from build123d import *

# Parameters (mm, degrees)
F0_R      = 10
F1_DEPTH  = 70
F1_TAPER  = -5
F2_R      = 8
F3_R      = 10
F3_R_2    = 7.5
F1_FACE_R = 10
F4_DEPTH  = 25


with BuildPart() as f1:
    # F0 (on Front) → F1 (new body)
    with BuildSketch(Plane.XZ):
        Circle(F0_R)
    extrude(amount=F1_DEPTH, taper=F1_TAPER)

    # F2
    f2_edges = [f1.edges().sort_by_distance(p)[0] for p in [
        (-16.124206, -70, 0),
    ]]
    fillet(f2_edges, radius=F2_R)

    # F3 (on face) + F1_face (on face) → F4 (join)
    with BuildSketch(Plane(origin=(0, 0, 0), x_dir=(-1, 0, 0), z_dir=(0, 1, 0))):
        Circle(F3_R)
        Circle(F3_R_2, mode=Mode.SUBTRACT)
    with BuildSketch(Plane(origin=(0, 0, 0), x_dir=(1, 0, 0), z_dir=(0, 1, 0))):
        Circle(F1_FACE_R)
    extrude(amount=F4_DEPTH)


solid = f1.part
CAD build for the part. Positions are in the model's coordinates, mm. Coordinates: 2 decimals unless noted, no trailing zeros. Loops run counter-clockwise (first coordinate to the right, second up) from the corner with the lowest first, then second, coordinate; pieces in that order, holes last. Notation, with made-up numbers: (-10, 37) - (21, 37) arc R18 ccw to (21, 68) - close; hole circle Ø8 at (81, 5). An arc over 180 degrees is marked (long way). Write item = value, one per line. Start each with the question number.
Q1. Cut at A-A, the plane y = 7. List the corners of the cut face in (x, z).
Q2. Flat gauge pins, fed straight in: pin 1 Ø2 at (y, z) = (-29.5, 1) entering from +X; pin 2 Ø1 at (x, y) = (2.5, -20.5) entering from +Z; pin 3 Ø3 at (x, y) = (-11, -5) entering from +Z. Where does each tip first touch, or does it go through?
Q3. Pull direction Z, two halves, no side cores. Call faces 1 (the cylindrical face through (2.17, 12.32, -9.76)), 2 (the flat face through (0, 25, 0)): pulls with the +Z half, pulls with the -Z half, needs draft (parallel to the pull), parting line crosses it, or undercut.
Q4. Drill centre lines: L1, parallel to Z at x = 0, y = 19; L2, parallel to Y at x = -6, z = -5.5; L3, parallel to X at y = -23.5, z = -10. Where is each one in solid material? Low to high.
Computed:
q1.outline = circle Ø20 at (0, 0)
q2.pin_1 = 12.65
q2.pin_2 = 11.63
q2.pin_3 = 4.34
q3.face_1 = parting line crosses it
q3.face_2 = needs draft
q4.L1 = -10 to 10
q4.L2 = -69.97 to 25
q4.L3 = -6.73 to 6.73
